Read the model definition and answer for the solid it produces. Units are mm, in the model's axes. Face numbers are marked on the shaded views. Coordinates: 2 decimals unless noted, no trailing zeros. Loops run counter-clockwise (first coordinate to the right, second up) from the corner with the lowest first, then second, coordinate; pieces in that order, holes last. Notation, with made-up numbers: M 56,-27.75 L 115,-27.75 A11 ccw 115,-23.75 Z; hole C 88,55.5 d7. An arc over 180 degrees is marked long. Use one line per item in the form item = value. Start each with the question number.
1. For a pull along Z with two mould halves and no side action, classify the marked faces 1 and 2 as released by +Z, released by -Z, zero draft, split by the parting line, or undercut.
2. Flat-ended cylindrical pins translate along their axes: pin 1 (3 mm diameter, centred on y = 20, z = -710.5, fed in from +X); pin 2 (10 mm diameter, centred on x = -11.5, z = 486, fed in from +Y); pin 3 (5 mm diameter, centred on x = -5.5, z = 298, fed in from +Y). Find the tip coordinate at first contact, or state that the pin passes through.
3. Find the intervals of material crossed by probe 1 along Y at (x, z) = (0, 283.5); probe 2 along Y at (x, z) = (4, -330.5); probe 3 along X at (y, z) = (-20.5, 51), in increasing order. Write a range as [from, to].
4. The part is cut by section C-C (z = 355). Give the vertices of the cut face in (x, y), plus the area to 3 significant figures.
5. The part is cut by section A-A (x = 0). Give the vertices of the cut face in (y, z).
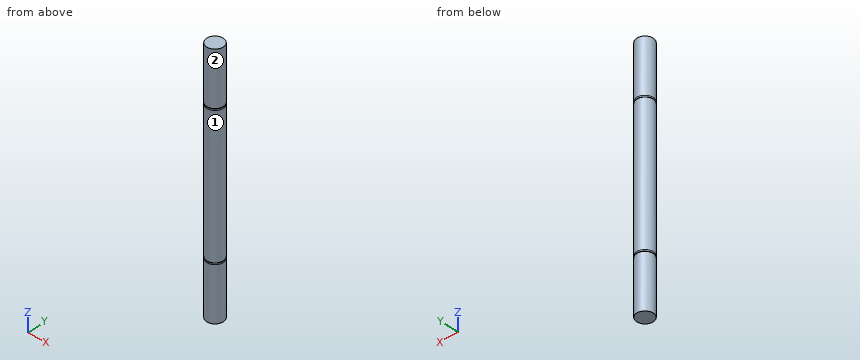
from build123d import *

# Parameters (mm, degrees)
F0_R     = 60
F1_DEPTH = 900
F4_R     = 62.5
F4_R_2   = 60
F5_DEPTH = 10


# Not quite as in the source:
# - a pattern or mirror of a feature is missing from the dataset's text; its kind, count and spacing are read off the source's solid


with BuildPart() as f1:
    # F0 (on Top) → F1 (new body)
    with BuildSketch(Plane.XY):
        Circle(F0_R)
    extrude(amount=F1_DEPTH)

    # F2: F1 across plane


with BuildPart() as f1_1:
    add(f1.part)
    add(f1.part.mirror(Plane.XY))

    # F4 (on offset) → F5 (join)
    with BuildSketch(Plane.XY.offset(500)):
        Circle(F4_R)
        Circle(F4_R_2, mode=Mode.SUBTRACT)
    f5 = extrude(amount=F5_DEPTH)

    # F5_copies: F5 across plane
    add(f5.mirror(Plane(origin=(0, 0, 0), x_dir=(-1, 0, 0), z_dir=(0, 0, -1))))


solid = f1_1.part
Computed values:
q1.face_1 = undercut
q1.face_2 = zero draft
q2.pin_1 = 57.08
q2.pin_2 = 59.65
q2.pin_3 = 59.92
q3.probe_1 = [-60, 60]
q3.probe_2 = [-59.87, 59.87]
q3.probe_3 = [-56.39, 56.39]
q4.outline = C 0,0 d120
q4.area = 11,300 mm²
q5.outline = M -62.5,-510 L -60,-510 L -60,-900 L 60,-900 L 60,-510 L 62.5,-510 L 62.5,-500 L 60,-500 L 60,500 L 62.5,500 L 62.5,510 L 60,510 L 60,900 L -60,900 L -60,510 L -62.5,510 L -62.5,500 L -60,500 L -60,-500 L -62.5,-500 Z
